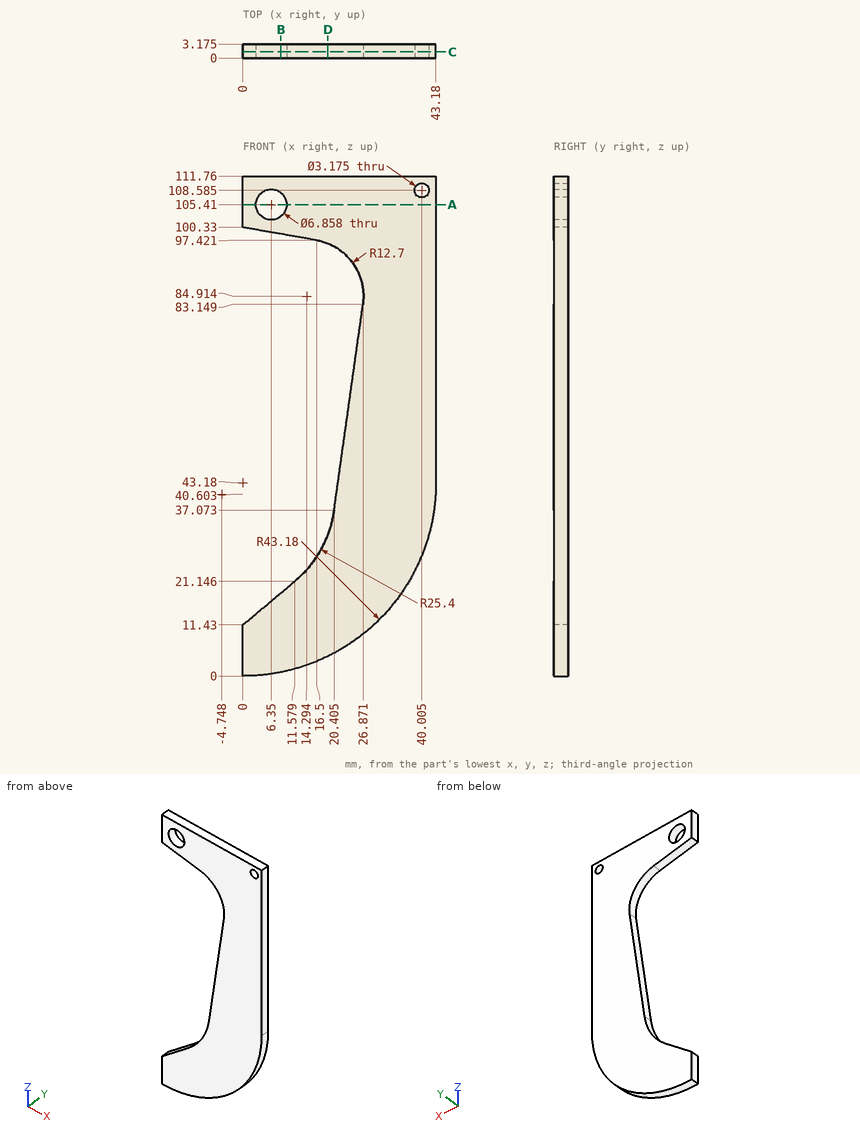
Can you work these out from the drawing? Everything is in mm from the part's minimum corner. Coordinates: 2 decimals unless noted, no trailing zeros. Loops run counter-clockwise (first coordinate to the right, second up) from the corner with the lowest first, then second, coordinate; pieces in that order, holes last.
1) For pin 1 (1.5 mm diameter, centred on x = 9, y = 1.5, fed in from -Z) (1 decimal); pin 2 (5 mm diameter, centred on x = 40.005, z = 108.585, fed in from -Y); pin 3 (5.5 mm diameter, centred on x = 6.35, z = 105.41, fed in from +Y) (3 decimals), each with a flat end and sliding along its axis, tell me the tip position at first contact or that it passes through.
2) Imagine slicing it at B-B on x = 8.5. List the corners of the cut face in (y, z) for me (1 decimal).
3) I need wall thicknesses on probe 1 along Z at (x, y) = (8, 0.65) (1 decimal); probe 2 along X at (y, z) = (0.65, 105.41); probe 3 along X at (y, z) = (0.7, 107.5) (1 decimal). Which ranges of each line are inside material? Lowest first, please.
4) Imagine slicing it at C-C on y = 1.4. State how many separate pieces and enclosed holes the cut face has, plus the area to 3 significant figures.
5) Imagine slicing it at D-D on x = 19. List the corners of the cut face in (y, z) for me (1 decimal), plus the area to 3 significant figures.
6) Imagine slicing it at A-A on z = 105.41. List the corners of the cut face in (x, y) for me (1 decimal), plus the area to 3 significant figures.
Completed:
1. pin 1: stops at z = 0.8
1. pin 2: stops at y = 0
1. pin 3: passes through
2. outline: (0, 0.8) - (3.2, 0.8) - (3.2, 18.6) - (0, 18.6) - close; (0, 98.8) - (3.2, 98.8) - (3.2, 102.7) - (0, 102.7) - close; (0, 108.1) - (3.2, 108.1) - (3.2, 111.8) - (0, 111.8) - close
3. probe 1: z = 0.7 to 18.1, 98.9 to 102.4, 108.4 to 111.8
3. probe 2: x = 0 to 2.92, 9.78 to 43.18
3. probe 3: x = 0 to 3.6, 9.1 to 38.8, 41.2 to 43.2
4. separate pieces: 1
4. enclosed holes: 2
4. area: 2,580 mm2
5. outline: (0, 4.4) - (3.2, 4.4) - (3.2, 31.6) - (0, 31.6) - close; (0, 96.7) - (3.2, 96.7) - (3.2, 111.8) - (0, 111.8) - close
5. area: 134 mm2
6. outline: (0, 0) - (2.9, 0) - (2.9, 3.2) - (0, 3.2) - close; (9.8, 0) - (43.2, 0) - (43.2, 3.2) - (9.8, 3.2) - close
6. area: 115 mm2
